Read the model definition and answer for the solid it produces. Units are mm, in the model's axes. Give positions to 0.01 mm unless a question says otherwise; leave off trailing zeros. Write each loop counter-clockwise with the first axis right and the second up, starting at its lowest first coordinate (ties: lowest second). Pieces come first, ordered by that corner, then holes. Notation, with made-up numbers: M 17,-19.5 L 75,-19.5 A8 cw 75,-11.5 Z; hole C 68,-21.75 d2. An arc over 180 degrees is marked long. Put each result on its own line as item: value.
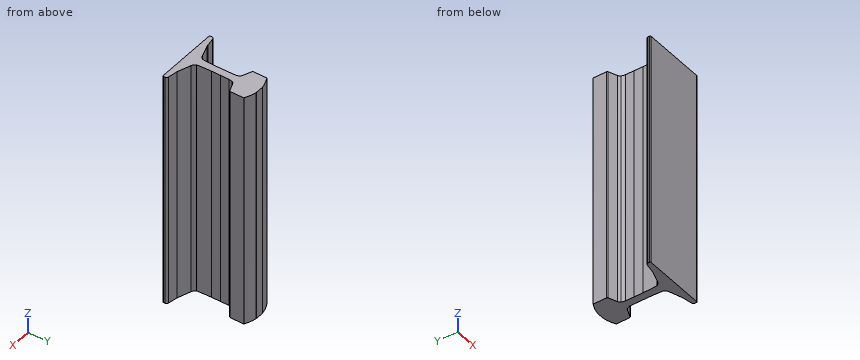
from build123d import *

# Parameters (mm, degrees)
BOSS_EXTRUDE1_DEPTH = 500


with BuildPart() as part:
    # Sketch3 → Boss-Extrude1 (new body)
    with BuildSketch(Plane.XY):
        with BuildLine():
            Line((0, 0), (-66, 0))
            ThreePointArc((-66, 0), (-67.414213562, 0.585786438), (-68, 2))
            Line((-68, 2), (-68, 4.765190248))
            ThreePointArc((-68, 4.765190248), (-66.815034418, 7.997142041), (-63.821795043, 9.697193178))
            Line((-63.821795043, 9.697193178), (-45.627404821, 12.72883365))
            ThreePointArc((-45.627404821, 12.72883365), (-44.016636876, 13.065865401), (-42.439030045, 13.534182026))
            Line((-42.439030045, 13.534182026), (-16.479262031, 22.417915838))
            ThreePointArc((-16.479262031, 22.417915838), (-12.091385863, 24.966143716), (-9.013249079, 29))
            ThreePointArc((-9.013249079, 29), (-8.065943267, 44.487135998), (-7.75, 60))
            Line((-7.75, 60), (-7.75, 79))
            ThreePointArc((-7.75, 79), (-7.803158877, 88.000627905), (-7.962628091, 97))
            ThreePointArc((-7.962628091, 97), (-8.43329292, 101.07664564), (-9.636561641, 105))
            ThreePointArc((-9.636561641, 105), (-11.41229559, 107.653272086), (-14.084201862, 109.400842023))
            Line((-14.084201862, 109.400842023), (-32.238737772, 116.616858833))
            ThreePointArc((-32.238737772, 116.616858833), (-33.154913222, 117.352365228), (-33.5, 118.475424545))
            Line((-33.5, 118.475424545), (-33.5, 147.339300155))
            ThreePointArc((-33.5, 147.339300155), (-21.78437547, 152.590959224), (-9.379525087, 155.900863764))
            ThreePointArc((-9.379525087, 155.900863764), (-9.003111167, 155.954824325), (-8.623684969, 155.980022357))
            ThreePointArc((-8.623684969, 155.980022357), (0, 156.101961392), (8.623684969, 155.980022357))
            ThreePointArc((8.623684969, 155.980022357), (9.003111167, 155.954824325), (9.379525087, 155.900863764))
            ThreePointArc((9.379525087, 155.900863764), (21.78437547, 152.590959224), (33.5, 147.339300155))
            Line((33.5, 147.339300155), (33.5, 118.475424545))
            ThreePointArc((33.5, 118.475424545), (33.154913222, 117.352365228), (32.238737772, 116.616858833))
            Line((32.238737772, 116.616858833), (14.084201862, 109.400842023))
            ThreePointArc((14.084201862, 109.400842023), (11.41229559, 107.653272086), (9.636561641, 105))
            ThreePointArc((9.636561641, 105), (8.43329292, 101.07664564), (7.962628091, 97))
            ThreePointArc((7.962628091, 97), (7.803158877, 88.000627905), (7.75, 79))
            Line((7.75, 79), (7.75, 60))
            ThreePointArc((7.75, 60), (8.065943267, 44.487135998), (9.013249079, 29))
            ThreePointArc((9.013249079, 29), (12.091385863, 24.966143716), (16.479262031, 22.417915838))
            Line((16.479262031, 22.417915838), (44, 12.999999996))
            Line((44, 12.999999996), (63.821795043, 9.697193178))
            ThreePointArc((63.821795043, 9.697193178), (66.815034418, 7.997142041), (68, 4.765190248))
            Line((68, 4.765190248), (68, 2))
            ThreePointArc((68, 2), (67.414213562, 0.585786438), (66, 0))
            Line((66, 0), (0, 0))
        make_face()
    extrude(amount=BOSS_EXTRUDE1_DEPTH)


solid = part.part
(1) Straight lines are drawn through the part: line 1 along X through (y, z) = (82, 243); line 2 along Y through (x, z) = (1.5, 119); line 3 along Y through (x, z) = (-7.5, 442.5). For each, find the intervals that lie inside material, in ascending order. Write a range as from..to.
Result:
line 1: x = -7.76..7.76
line 2: y = 0..156.1
line 3: y = 0..156.01
(2) Section A-A on x = 26 is taken. Determine the outline of the cut face in (y, z), and give its area (3 significant figures).
Result:
outline: M 0,0 L 19.16,0 L 19.16,500 L 0,500 Z; M 114.14,0 L 150.96,0 L 150.96,500 L 114.14,500 Z
area: 28,000 mm²
(3) Given pin 1 Ø9.5 at (y, z) = (65, 318.5) entering from +X; pin 2 Ø12 at (x, z) = (22.5, 247.5) entering from +Y; pin 3 Ø8.5 at (y, z) = (135, 158) entering from +X, each flat-ended and moving along its own axis, determine where each tip first touches the part or whether it passes through.
Result:
pin 1: stops at x = 7.75
pin 2: stops at y = 154.26
pin 3: stops at x = 33.5
(4) Section C-C on x = -51 is taken. Determine the outline of the cut face in (y, z).
Result:
outline: M 0,0 L 11.83,0 L 11.83,500 L 0,500 Z
(5) Section B-B on y = 141 is taken. Determine the outline of the cut face in (x, z).
Result:
outline: M -33.5,0 L 33.5,0 L 33.5,500 L -33.5,500 Z
